from build123d import *

# Parameters (mm, degrees)
SKETCH1_R           = 1.5
BOSS_EXTRUDE1_DEPTH = 3
LPATTERN1_COUNT     = 2
LPATTERN1_PITCH     = 15
FILLET2_R           = 3
FILLET3_R           = 3
SKETCH2_W           = 14.977515773
SKETCH2_H           = 2.058823846
BOSS_EXTRUDE2_DEPTH = 15
SKETCH3_R           = 3
SKETCH3_R_2         = 1.5
BOSS_EXTRUDE3_DEPTH = 4
LPATTERN2_COUNT     = 2
LPATTERN2_PITCH     = 8


with BuildPart() as part:
    # Sketch1 → Boss-Extrude1 (new body)
    with BuildSketch(Plane.XY):
        with BuildLine():
            Line((0, 0), (30, 0))
            ThreePointArc((30, 0), (21.213203436, -21.213203436), (0, -30))
            Line((0, -30), (0, 0))
        make_face()
        with Locations((3, -26)):
            Circle(SKETCH1_R, mode=Mode.SUBTRACT)
        with Locations((3, -3)):
            Circle(SKETCH1_R, mode=Mode.SUBTRACT)
        with BuildLine():
            ThreePointArc((21.329556778, -5.505463694), (17.394405246, -14.621148722), (9.313112731, -20.38949705))
            ThreePointArc((9.313112731, -20.38949705), (8.415027516, -22.311330275), (10.336860742, -23.20941549))
            ThreePointArc((10.336860742, -23.20941549), (19.728633123, -16.505659326), (24.301917337, -5.911755103))
            ThreePointArc((24.301917337, -5.911755103), (23.018882762, -4.222429119), (21.329556778, -5.505463694))
        make_face(mode=Mode.SUBTRACT)
    extrude(amount=BOSS_EXTRUDE1_DEPTH)


with BuildPart() as lpattern1_1:
    # LPattern1: pattern copy
    add(part.part.moved(Location(Vector(0, 0, 1) * (1 * LPATTERN1_PITCH))))

    # Fillet3
    fillet3_edges = [lpattern1_1.edges().sort_by_distance(p)[0] for p in [
        (0, 0, 16.5),
        (30, 0, 16.5),
        (0, -30, 16.5),
    ]]
    fillet(fillet3_edges, radius=FILLET3_R)


with BuildPart() as part_1:
    add(part.part)

    # Fillet2
    fillet2_edges = [part_1.edges().sort_by_distance(p)[0] for p in [
        (0, 0, 1.5),
        (30, 0, 1.5),
        (0, -30, 1.5),
    ]]
    fillet(fillet2_edges, radius=FILLET2_R)

    add(lpattern1_1.part)  # Boss-Extrude2 merges LPattern1_1
    # Sketch2 → Boss-Extrude2 (add)
    with BuildSketch(Plane.XY.offset(3)):
        with Locations((19.344057843, -1.029411923)):
            Rectangle(SKETCH2_W, SKETCH2_H)
    extrude(amount=BOSS_EXTRUDE2_DEPTH)

    # Sketch3 → Boss-Extrude3 (add)
    with BuildSketch(Plane(origin=(0, 0, 15), x_dir=(-1, 0, 0), z_dir=(0, 0, -1))):
        with Locations((-3, -26)):
            Circle(SKETCH3_R)
        with Locations((-3, -26)):
            Circle(SKETCH3_R_2, mode=Mode.SUBTRACT)
    boss_extrude3 = extrude(amount=BOSS_EXTRUDE3_DEPTH)

    # LPattern2: Boss-Extrude3 ×2
    with Locations(*[(0, 0, -i * LPATTERN2_PITCH) for i in range(1, LPATTERN2_COUNT)]):
        add(boss_extrude3)


solid = part_1.part
Part model, mm, in its own coordinate system. A direction names the side the tool comes from. Round coordinates to 2 decimals unless told otherwise and drop trailing zeros. Write each loop counter-clockwise with the first axis right and the second up, starting at its lowest first coordinate (ties: lowest second). Pieces come first, ordered by that corner, then holes. Notation, with made-up numbers: (-7.5, 74) - (45.5, 74) arc R34 cw to (45.5, 105) - close; hole circle Ø5 at (-36.5, 54). An arc over 180 degrees is marked (long way). Use CSV: the item, a comma, the result in double quotes.
Item 1: Flat gauge pins, fed straight in: P1, Ø2.5, axis at y = -1, z = 6.5, coming from the -X side; P2, Ø2.5, axis at x = 3, y = -26, coming from the +Z side; P3, Ø2, axis at x = 19.5, z = 9.5, coming from the -Y side; P4, Ø1.6, axis at y = -1.5, z = 6, coming from the +X side. Where does each tip first touch, or does it go through?
Results list:
P1,"stops at x = 11.86"
P2,"passes through"
P3,"stops at y = -2.06"
P4,"stops at x = 26.83"
Item 2: Wall check: L1, parallel to Y at x = 3, z = 2.25; L2, parallel to Z at x = 6.75, y = -27; L3, parallel to Z at x = 4.25, y = -27. Give the ranges that are in metal, low to high.
Results list:
L1,"y = -29.83 to -27.5, -24.5 to -4.5, -1.5 to 0"
L2,"z = 0 to 3, 15 to 18"
L3,"z = 0 to 7, 11 to 18"
Item 3: Slice it at C-C, the plane x = 21.75. Write the cut outline in (y, z).
Results list:
outline,"(-20.66, 0) - (-13.52, 0) - (-13.52, 3) - (-20.66, 3) - close; (-20.66, 15) - (-13.52, 15) - (-13.52, 18) - (-20.66, 18) - close; (-4.65, 0) - (0, 0) - (0, 18) - (-4.65, 18) - (-4.65, 15) - (-2.06, 15) - (-2.06, 3) - (-4.65, 3) - close"
Item 4: Tool access for faces 5 (the cylindrical face through (17.482, -14.511, 16.479)), 6 (the cylindrical face through (5.4, -27.8, 13)), 7 (the cylindrical face through (21.412, -21.012, 1.479)): list every direction of +Z, -Z, +X, -X, +Y, -Y with a clear straight run to the whole face (end or side of a thin tool).
Results list:
face 5,"+Z, -Z"
face 6,"none"
face 7,"+Z, -Z, +X, -Y"
Item 5: Slice it at A-A, the plane z = 4.25. Write the cut outline in (x, y).
Results list:
outline,"circle Ø6 at (3, -26); (11.86, -2.06) - (26.83, -2.06) - (26.83, 0) - (11.86, 0) - close; hole circle Ø3 at (3, -26)"
Item 6: Slice it at D-D, the plane z = 16. Write the cut outline in (x, y), then the cut area to 3 significant figures.
Results list:
outline,"(0, -26.83) arc R3 ccw to (3.33, -29.81) arc R30 ccw to (29.81, -3.33) arc R3 ccw to (26.83, 0) - (3, 0) arc R3 ccw to (0, -3) - close; hole circle Ø3 at (3, -26); hole circle Ø3 at (3, -3); hole (9.31, -20.39) arc R1.5 ccw to (10.34, -23.21) arc R21.5 ccw to (24.3, -5.91) arc R1.5 ccw to (21.33, -5.51) arc R18.5 cw to start"
area,"614 mm²"
Item 7: Pull direction Z, two halves, no side cores. Call faces 1 (the flat face through (12, -11, 15)), 2 (the flat face through (12, -11, 18)), 3 (the flat face through (1.7, -27.3, 7)), 4 (the cylindrical face through (19.63, -16.63, 16.48)): pulls with the +Z half, pulls with the -Z half, needs draft (parallel to the pull), parting line crosses it, or undercut.
Results list:
face 1,"undercut"
face 2,"pulls with the +Z half"
face 3,"undercut"
face 4,"needs draft"
Item 8: Slice it at B-B, the plane y = -7.5. Write the cut outline in (x, z).
Results list:
outline,"(0, 0) - (20.94, 0) - (20.94, 3) - (0, 3) - close; (0, 15) - (20.94, 15) - (20.94, 18) - (0, 18) - close; (24.02, 0) - (29.05, 0) - (29.05, 3) - (24.02, 3) - close; (24.02, 15) - (29.05, 15) - (29.05, 18) - (24.02, 18) - close"
